Check sheet for the drawn part. Datum: minimum x, y, z corner. Units: mm. Coordinates: 2 decimals unless noted, no trailing zeros. Order: outer loops, then holes, each group sorted by start corner. A loop starts at its lowest first (then second) coordinate and runs counter-clockwise, first axis right, second up. Notation, with made-up numbers: (63.5, 56.25) - (122.5, 56.25) arc R18 ccw to (122.5, 77.25) - close; hole circle Ø9 at (36.5, 2.5). An arc over 180 degrees is marked (long way). Put each result on its own line as item: value.
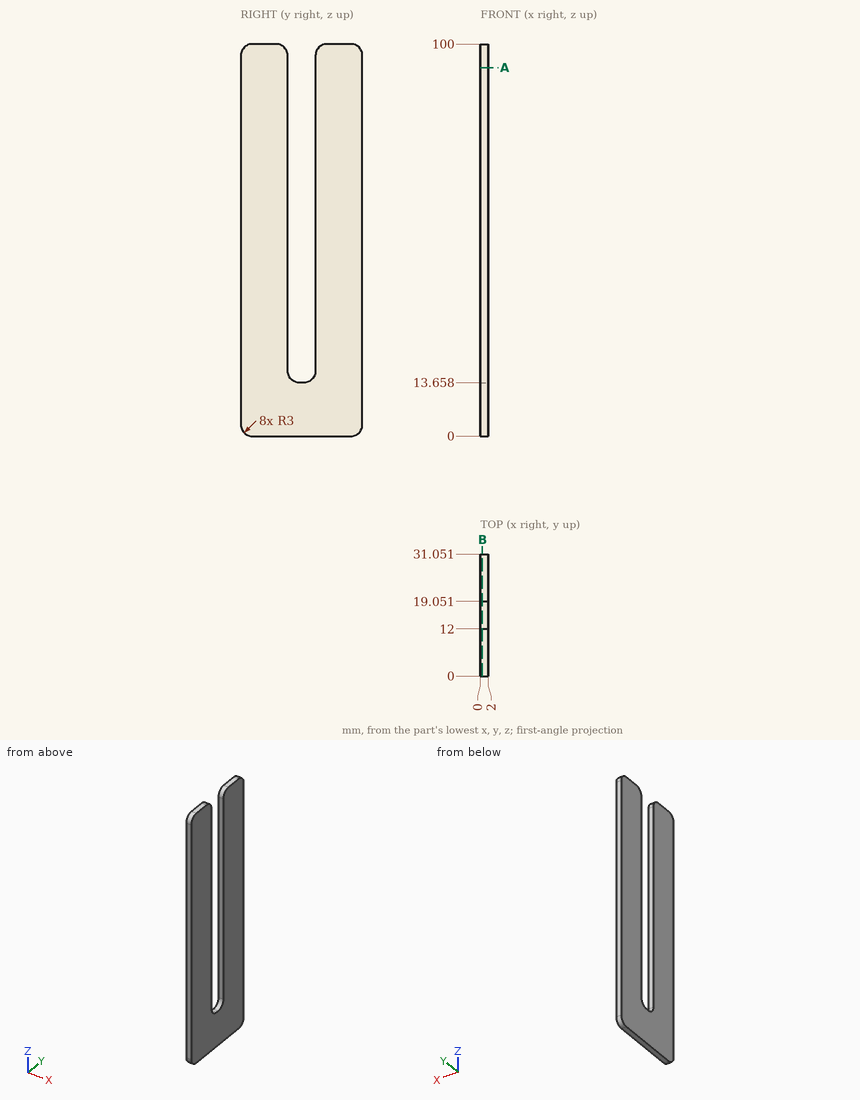
Q1. Thickness scan on L1, parallel to Y at x = 0.55, z = 27.5; L2, parallel to Z at x = 0.65, y = 11 (1 decimal); L3, parallel to Z at x = 1.55, y = 30. Record the ranges inside material, lowest first. Write a range as [from, to].
Answer block:
L1: y = [0, 12], [19.05, 31.05]
L2: z = [0, 99.2]
L3: z = [0.72, 99.28]
Q2. Section check B-B on x = 0.5. Record the boundary of the cut face in (y, z), then the cut area to 3 significant figures.
Answer block:
outline: (0, 3) arc R3 ccw to (3, 0) - (28.05, 0) arc R3 ccw to (31.05, 3) - (31.05, 97) arc R3 ccw to (28.05, 100) - (22.05, 100) arc R3 ccw to (19.05, 97) - (19.05, 16.66) arc R3 cw to (16.05, 13.66) - (15, 13.66) arc R3 cw to (12, 16.66) - (12, 97) arc R3 ccw to (9, 100) - (3, 100) arc R3 ccw to (0, 97) - close
area: 2,490 mm^2
Q3. Section check A-A on z = 94. Record the boundary of the cut face in (x, y), then the cut area to 3 significant figures.
Answer block:
outline: (0, 0) - (2, 0) - (2, 12) - (0, 12) - close; (0, 19.05) - (2, 19.05) - (2, 31.05) - (0, 31.05) - close
area: 48.0 mm^2
Q4. Depth check by flat-ended pin: pin 1 Ø0.5 at (x, y) = (0.5, 15.5) entering from +Z. Enter the tip coordinate at first touch or a pass-through.
Answer block:
pin 1: stops at z = 13.66
